Input: part model. Units: mm. Frame: model coordinates. Give positions to 0.01 mm unless a question says otherwise; leave off trailing zeros. Loops run counter-clockwise (first coordinate to the right, second up) from the corner with the lowest first, then second, coordinate; pieces in that order, holes last. Notation, with made-up numbers: (-1.5, 39.5) - (20.5, 39.5) arc R18 ccw to (20.5, 64.5) - close; hole circle Ø8 at (53, -40). An arc over 180 degrees is marked (long way). Answer as a JSON object with one key per item and string values. Group by question number.
(1) Section query B-B (x = -16). Return loops of the section in (y, z), plus the area to 3 significant figures.
(2) Section query C-C (y = 8). Return loops of the section in (x, z), plus the area to 3 significant figures.
(3) Section query A-A (z = 16). Return loops of the section in (x, y), plus the area to 3 significant figures.
(4) Pin query (flat end, axial travel): P1, Ø0.9, axis at y = 5, z = 16.5, coming from the +X side; P2, Ø1.8, axis at x = 16, y = 5, coming from the +Z side; P3, Ø1.5, axis at y = 5.5, z = -16, coming from the -X side. Return the tip coordinate at first contact, or that it passes through.
(5) Material intervals for L1, parallel to Z at x = -30.5, y = 4.75; L2, parallel to Y at x = 36, z = 16; L3, parallel to X at y = 5.25, z = -33, sorted ascending.
Autodesk Inventor part; units mm, degrees
ref_plane "YZ Plane" through (0, 0, 0) normal (1, 0, 0) x (0, 1, 0)
ref_plane "XZ Plane" through (0, 0, 0) normal (0, 1, 0) x (-1, 0, 0)
ref_plane "XY Plane" through (0, 0, 0) normal (0, 0, 1) x (1, 0, 0)
sketch "Эскиз1" plane through (0, 0, 0) normal (0, 1, 0) x (-1, 0, 0)
  circle A0 centre (35.3553, 35.3553) radius 2
  circle A1 centre (-35.3553, 35.3553) radius 2
  circle A2 centre (-35.3553, -35.3553) radius 2
  circle A3 centre (35.3553, -35.3553) radius 2
  line L0 (-40, 40) -> (40, 40)
  line L1 (40, 40) -> (40, -40)
  line L2 (40, -40) -> (-40, -40)
  line L3 (-40, -40) -> (-40, 40)
  line L4 (-40, 40) -> (40, -40) construction
  line L5 (40, 40) -> (-40, -40) construction
  line L6 (35.3553, 35.3553) -> (0, 0) construction
  line L7 (0, 0) -> (0, 4.1405) construction
  dimension "d0" = 4
  dimension "d1" = 50
  dimension "d4" = 360
  dimension "d6" = 80
  dimension "d7" = 80
  dimension "d17" = 45
extrude "Выдавливание1" add sketch "Эскиз1" along normal blind 10
sketch "Эскиз2" plane through (0, 10, 0) normal (0, 1, 0) x (1, 0, 0)
  circle A0 centre (-35.3553, -35.3553) radius 2
  circle A1 centre (-35.3553, -35.3553) radius 7.5
  point P0 (0, 0)
  dimension "d10" = 15
extrude "Выдавливание2" cut sketch "Эскиз2" against normal blind 5
pattern_circular "Круговой массив1" count 4 over 360 about axis through (0, -10, 0) along (0, 1, 0) of "Выдавливание2"
fillet "Сопряжение1" radius 4.75 12 edges at (29.4666, 7.5, 40) (40, 7.5, 29.4666) (40, 7.5, -29.4666) (29.4666, 7.5, -40) (-29.4666, 7.5, -40) (-40, 7.5, -29.4666) (-40, 7.5, 29.4666) (-29.4666, 7.5, 40) (-40, 2.5, 40) (40, 2.5, 40) (40, 2.5, -40) (-40, 2.5, -40)
sketch "Эскиз3" plane through (-35.25, 0, 40) normal (0, 0, 1) x (1, 0, 0)
  circle A0 centre (19.25, 5) radius 1.5
  circle A1 centre (51.25, 5) radius 1.5
  line L0 (0, 0) -> (70.5, 0)
  line L1 (35.25, 0) -> (35.25, 5.0167)
  dimension "d18" = 3
  dimension "d19" = 3
  dimension "d20" = 5
  dimension "d21" = 16
extrude "Выдавливание3" cut sketch "Эскиз3" against normal blind 10
pattern_circular "Круговой массив2" count 4 over 360 about axis through (0, -10, 0) along (0, 1, 0) of "Выдавливание3"
sketch "Эскиз4" plane through (-35.25, 0, 40) normal (0, 0, 1) x (1, 0, 0)
  circle A0 centre (51.25, 5) radius 1.5
  circle A1 centre (19.25, 5) radius 1.5
  line L0 (70.5, 5) -> (70.5, 0)
  line L1 (70.5, 5) -> (58.3558, 5)
  line L2 (58.3558, 10) -> (58.3558, 5)
  line L3 (12.1442, 10) -> (58.3558, 10)
  line L4 (12.1442, 5) -> (12.1442, 10)
  line L5 (12.1442, 5) -> (0, 5)
  line L6 (0, 0) -> (0, 5)
  line L7 (0, 0) -> (70.5, 0)
  point P0 (35.25, 0)
properties part number "KB33-046-009 - Колпак лидара"
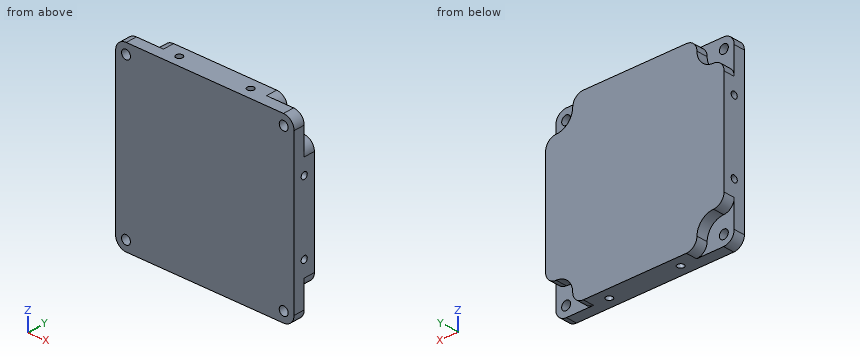
Recorded:
{
 "1": {"outline": "(0, -40) - (3.5, -40) - (3.5, -30) - (6.5, -30) - (6.5, -40) - (10, -40) - (10, 40) - (6.5, 40) - (6.5, 30) - (3.5, 30) - (3.5, 40) - (0, 40) - close", "area": "740 mm^2"},
 "2": {"outline": "(-40, -23.11) arc R4.75 ccw to (-35.29, -27.86) arc R7.5 cw to (-27.86, -35.29) arc R4.75 ccw to (-23.11, -40) - (23.11, -40) arc R4.75 ccw to (27.86, -35.29) arc R7.5 cw to (35.29, -27.86) arc R4.75 ccw to (40, -23.11) - (40, 23.11) arc R4.75 ccw to (35.29, 27.86) arc R7.5 cw to (27.86, 35.29) arc R4.75 ccw to (23.11, 40) - (-23.11, 40) arc R4.75 ccw to (-27.86, 35.29) arc R7.5 cw to (-35.29, 27.86) arc R4.75 ccw to (-40, 23.11) - close", "area": "5,820 mm^2"},
 "3": {"outline": "(-40, 0) - (40, 0) - (40, 3.5) - (30, 3.5) - (30, 6.5) - (40, 6.5) - (40, 10) - (-40, 10) - (-40, 6.5) - (-30, 6.5) - (-30, 3.5) - (-40, 3.5) - close", "area": "740 mm^2"},
 "4": {"P1": "stops at x = 30", "P2": "stops at z = 30", "P3": "stops at x = -30"},
 "5": {"L1": "z = -40 to -17.48, -14.52 to 14.52, 17.48 to 40", "L2": "y = 0 to 3.5, 6.5 to 10", "L3": "x = -28.23 to -17.48, -14.52 to 14.52, 17.48 to 28.23"}
}
